```python
from build123d import *

# Parameters (mm, degrees)
SKETCH_2_R      = 2.5
EXTRUDE_1_DEPTH = 150


with BuildPart() as part:
    # 草图2 → 凸台-拉伸1 (new body)
    with BuildSketch(Plane(origin=(0, 0, 0), x_dir=(1, 0, 0), z_dir=(0, 1, 0))):
        with BuildLine():
            Line((-2.839339828, -3.9), (-5.5, -6.560660172))
            Line((-5.5, -6.560660172), (-5.5, -8.2))
            Line((-5.5, -8.2), (-3.1, -8.2))
            Line((-3.1, -8.2), (-3.1, -10))
            Line((-3.1, -10), (-8.5, -10))
            ThreePointArc((-8.5, -10), (-9.560660172, -9.560660172), (-10, -8.5))
            Line((-10, -8.5), (-10, -3.1))
            Line((-10, -3.1), (-8.2, -3.1))
            Line((-8.2, -3.1), (-8.2, -5.5))
            Line((-8.2, -5.5), (-6.560660172, -5.5))
            Line((-6.560660172, -5.5), (-3.9, -2.839339828))
            Line((-3.9, -2.839339828), (-3.9, 2.839339828))
            Line((-3.9, 2.839339828), (-6.560660172, 5.5))
            Line((-6.560660172, 5.5), (-8.2, 5.5))
            Line((-8.2, 5.5), (-8.2, 3.1))
            Line((-8.2, 3.1), (-10, 3.1))
            Line((-10, 3.1), (-10, 8.5))
            ThreePointArc((-10, 8.5), (-9.560660172, 9.560660172), (-8.5, 10))
            Line((-8.5, 10), (-3.1, 10))
            Line((-3.1, 10), (-3.1, 8.2))
            Line((-3.1, 8.2), (-5.5, 8.2))
            Line((-5.5, 8.2), (-5.5, 6.560660172))
            Line((-5.5, 6.560660172), (-2.839339828, 3.9))
            Line((-2.839339828, 3.9), (2.839339828, 3.9))
            Line((2.839339828, 3.9), (5.5, 6.560660172))
            Line((5.5, 6.560660172), (5.5, 8.2))
            Line((5.5, 8.2), (3.1, 8.2))
            Line((3.1, 8.2), (3.1, 10))
            Line((3.1, 10), (8.5, 10))
            ThreePointArc((8.5, 10), (9.560660172, 9.560660172), (10, 8.5))
            Line((10, 8.5), (10, 3.1))
            Line((10, 3.1), (8.2, 3.1))
            Line((8.2, 3.1), (8.2, 5.5))
            Line((8.2, 5.5), (6.560660172, 5.5))
            Line((6.560660172, 5.5), (3.9, 2.839339828))
            Line((3.9, 2.839339828), (3.9, -2.839339828))
            Line((3.9, -2.839339828), (6.560660172, -5.5))
            Line((6.560660172, -5.5), (8.2, -5.5))
            Line((8.2, -5.5), (8.2, -3.1))
            Line((8.2, -3.1), (10, -3.1))
            Line((10, -3.1), (10, -8.5))
            ThreePointArc((10, -8.5), (9.560660172, -9.560660172), (8.5, -10))
            Line((8.5, -10), (3.1, -10))
            Line((3.1, -10), (3.1, -8.2))
            Line((3.1, -8.2), (5.5, -8.2))
            Line((5.5, -8.2), (5.5, -6.560660172))
            Line((5.5, -6.560660172), (2.839339828, -3.9))
            Line((2.839339828, -3.9), (-2.839339828, -3.9))
        make_face()
        with Locations(Location((0, 0, 0), (0, 0, 270))):
            Circle(SKETCH_2_R, mode=Mode.SUBTRACT)
    extrude(amount=EXTRUDE_1_DEPTH)


solid = part.part
```
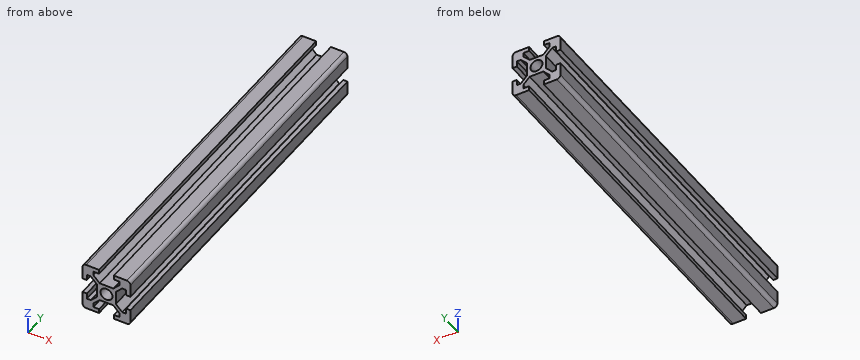
Design review of the part built by this model. Coordinates are the model's own, in mm. Coordinates: 2 decimals unless noted, no trailing zeros. Loops run counter-clockwise (first coordinate to the right, second up) from the corner with the lowest first, then second, coordinate; pieces in that order, holes last.
Q1. For pin 1 (3 mm diameter, centred on x = -0.5, y = 84, fed in from +Z); pin 2 (0.9 mm diameter, centred on y = 45, z = -9.5, fed in from +X); pin 3 (0.5 mm diameter, centred on y = 99.5, z = 9, fed in from -X), all flat-tipped, find the tip position at first contact; note any pin that passes through.
Reported:
pin 1: stops at z = 3.9
pin 2: stops at x = 9.9
pin 3: stops at x = -9.98
Q2. To check wall thickness, follow line 1 (Z direction, x = 4, y = 76); line 2 (X direction, y = 68.5, z = 5); line 3 (X direction, y = 87, z = 0). State the ranges of each line that lie inside material, in increasing order.
Reported:
line 1: z = -10 to -8.2, -5.06 to -2.94, 2.94 to 5.06, 8.2 to 10
line 2: x = -10 to -8.2, -6.06 to -3.94, 3.94 to 6.06, 8.2 to 10
line 3: x = -3.9 to -2.5, 2.5 to 3.9
Q3. We need section B-B on z = 0. State the section outline as (x, y) points.
Reported:
outline: (-3.9, 0) - (-2.5, 0) - (-2.5, 150) - (-3.9, 150) - close; (2.5, 0) - (3.9, 0) - (3.9, 150) - (2.5, 150) - close
Q4. We need section A-A on x = 0. State the section outline as (y, z) points, and give its area (3 significant figures).
Reported:
outline: (0, -3.9) - (150, -3.9) - (150, -2.5) - (0, -2.5) - close; (0, 2.5) - (150, 2.5) - (150, 3.9) - (0, 3.9) - close
area: 420 mm2
